Autodesk Inventor part; units mm, degrees
ref_plane "Płaszczyzna konstrukcyjna1" through (0, -12, 0) normal (0, 0, -1) x (-1, 0, 0)
ref_plane "Płaszczyzna konstrukcyjna2" through (0, -10, -2.2657) normal (1, 0, 0) x (0, 0, -1)
ref_plane "YZ Plane" through (0, 0, 0) normal (1, 0, 0) x (0, 1, 0)
sketch "Szkic1" plane through (0, 0, 0) normal (0, 1, 0) x (-1, 0, 0)
  circle A0 centre (0, 0) radius 12.5
  circle A1 centre (0, 0) radius 10
  dimension "d0" = 20
  dimension "d2" = 25
extrude "Wyciągnięcie proste1" add sketch "Szkic1" along normal blind 5
ref_plane "Płaszczyzna konstrukcyjna1" through (0, -12, 0) normal (0, 0, -1) x (-1, 0, 0)
sketch "Szkic5" plane through (0, -12, 0) normal (0, 0, -1) x (-1, 0, 0)
  line L0 (12.5, 17) -> (-12.5, 17)
  line L1 (0, 17) -> (-12.5, 17)
  line L2 (-12.5, 17) -> (-12.5, 19.375)
  line L3 (-12.5, 19.375) -> (0, 19.375)
  line L4 (0, 19.375) -> (0, 17)
  line L5 (0, 19.375) -> (-9.5, 19.375)
  line L6 (-9.5, 19.375) -> (-9.5, 21.875)
  line L7 (-9.5, 21.875) -> (0, 21.875)
  line L8 (0, 21.875) -> (0, 19.375)
  line L9 (0, 21.875) -> (-12.5, 21.875)
  line L10 (-12.5, 21.875) -> (-12.5, 24.25)
  line L11 (-12.5, 24.25) -> (0, 24.25)
  line L12 (0, 24.25) -> (0, 21.875)
  line L13 (0, 24.25) -> (-9.5, 24.25)
  line L14 (-9.5, 24.25) -> (-9.5, 26.75)
  line L15 (-9.5, 26.75) -> (0, 26.75)
  line L16 (0, 26.75) -> (0, 24.25)
  line L17 (0, 26.75) -> (-12.5, 26.75)
  line L18 (-12.5, 26.75) -> (-12.5, 29.125)
  line L19 (-12.5, 29.125) -> (0, 29.125)
  line L20 (0, 29.125) -> (0, 26.75)
  line L21 (0, 29.125) -> (-9.5, 29.125)
  line L22 (-9.5, 29.125) -> (-9.5, 31.625)
  line L23 (-9.5, 31.625) -> (0, 31.625)
  line L24 (0, 31.625) -> (0, 29.125)
  line L25 (0, 31.625) -> (-12.5, 31.625)
  line L26 (-12.5, 31.625) -> (-12.5, 34)
  line L27 (-12.5, 34) -> (0, 34)
  line L28 (0, 34) -> (0, 31.625)
  line L29 (-12.5, 12) -> (-12.5, 17) construction
  line L30 (-12.5, 12) -> (-12.5, 17) construction
  line L31 (-12.5, 12) -> (12.5, 12) construction
  point P0 (0, 12)
  dimension "d13" = 2.5
  dimension "d17" = 22
  dimension "d18" = 3
revolve "Obrót1" add sketch "Szkic5" angle 360 about axis through (0, 12.25, 0) along (0, -1, 0)
sketch "Szkic7" plane through (0, 19.625, 0) normal (0, -1, 0) x (1, 0, 0)
  circle A0 centre (0, 0) radius 9.5
  circle A1 centre (0, 9.5) radius 1.65
  circle A2 centre (0, 0) radius 10
  circle A3 centre (0, 0) radius 9.5
  circle A4 centre (-9.5, 0) radius 1.65
  circle A5 centre (0, -9.5) radius 1.65
  circle A6 centre (9.5, 0) radius 1.65
  circle A7 centre (6.7175, -6.7175) radius 0.9
  circle A8 centre (6.7175, 6.7175) radius 0.9
  circle A9 centre (-6.7175, 6.7175) radius 0.9
  circle A10 centre (-6.7175, -6.7175) radius 0.9
  line L0 (6.7175, 6.7175) -> (0, 0) construction
  line L1 (0, 0) -> (-6.7175, 6.7175) construction
  circle A11 centre (0, 0) radius 12.5 construction
  line L2 (0, 0) -> (-6.7175, -6.7175) construction
  line L3 (0, 0) -> (6.7175, -6.7175) construction
  line L4 (17.5, 0) -> (-17.5, 0) construction
  dimension "d23" = 45
  dimension "d24" = 45
  dimension "d25" = 3.3
  dimension "d47" = 1.8
extrude "Wyciągnięcie proste6" cut sketch "Szkic7" along normal up to surface (12.25 mm away) contours A0 A6 | A0 A6 A2 | A8 A0 | A0 A8 A2 | A6 A2 | A7 A2 A0 | A0 A7 | A2 A8 | A7 A2 | A1 A0 | A0 A1 A2 | A5 A2 A0 | A0 A5 | A2 A1 | A5 A2 | A9 A0 | A0 A9 A2 | A10 A2 A0 | A0 A10 | A2 A9 | A10 A2 | A4 A0 | A0 A4 A2 | A2 A4
sketch "Szkic8" plane through (0, -12, 0) normal (0, 0, -1) x (-1, 0, 0)
  line L0 (-1.65, 24.25) -> (1.65, 24.25)
  line L1 (-1.65, 29.125) -> (-1.65, 21.875)
  line L2 (1.65, 24.25) -> (-1.65, 24.25)
  line L3 (-1.65, 24.25) -> (-1.65, 26.751)
  line L4 (-1.65, 26.751) -> (1.65, 26.751)
  line L5 (1.65, 26.751) -> (1.65, 24.25)
  point P0 (0, 12)
  point P1 (-1.6438, 24.25)
  point P2 (1.6438, 24.25)
extrude "Wyciągnięcie proste7" cut sketch "Szkic8" along normal through all both and the other way through all
sketch "Szkic9" plane through (0, 5, 0) normal (0, -1, 0) x (1, 0, 0)
  line L0 (0, 0) -> (-3.4352, 0)
  line L1 (-3.4352, 0) -> (-3.4352, -2.2657)
  line L2 (-3.4352, -2.2657) -> (0, -2.2657)
  line L3 (0, -2.2657) -> (0, 0)
  dimension "d30" = 3.4352
  dimension "d31" = 2.2658
extrude "Wyciągnięcie proste8" add sketch "Szkic9" along normal blind 15
ref_plane "Płaszczyzna konstrukcyjna2" through (0, -10, -2.2657) normal (1, 0, 0) x (0, 0, -1)
sketch "Szkic10" plane through (0, -10, 0) normal (0, -1, 0) x (1, 0, 0)
  line L0 (0, 0) -> (-3.4352, 0)
  line L1 (-3.4352, -2.2657) -> (0, -2.2657)
  line L2 (0, 0) -> (-3.4352, 0)
  line L3 (-3.4352, 0) -> (-3.4352, -2.2657)
  line L4 (-3.4352, -2.2657) -> (0, -2.2657)
  line L5 (0, -2.2657) -> (0, 0)
extrude "Wyciągnięcie proste9" cut sketch "Szkic10" against normal up to surface (15 mm away)
sketch "Szkic11" plane through (0, -10, -2.2657) normal (1, 0, 0) x (0, 0, -1)
  line L0 (-3.9095, 22.25) -> (-3.9095, 24.75)
  line L1 (-0.622, 22.25) -> (-0.622, 24.75)
  line L2 (-3.9095, 22.25) -> (-0.622, 22.25)
  line L3 (-0.622, 22.25) -> (-0.622, 24.75)
  line L4 (-0.622, 24.75) -> (-3.9095, 24.75)
  line L5 (-3.9095, 24.75) -> (-3.9095, 22.25)
  point P0 (-2.2657, 10)
extrude "Wyciągnięcie proste10" cut sketch "Szkic11" along normal through all both and the other way through all
sketch "Szkic12" plane through (0, 22, 0) normal (0, 1, 0) x (1, 0, 0)
  line L0 (0, 0) -> (-4.4901, 4.4901) construction
  line L1 (0, 0) -> (0, 6.35) construction
  line L2 (0, 0) -> (-4.4901, -4.4901) construction
  line L3 (0, 0) -> (4.4901, -4.4901) construction
  line L4 (0, 0) -> (4.4901, 4.4901) construction
  circle A0 centre (0, 0) radius 6.35 construction
  circle A1 centre (0, 0) radius 12.5 construction
  point P0 (-4.4901, -4.4901)
  dimension "d48" = 45
  dimension "d49" = 12.7
hole "Otwór1" at (-4.4901, 22, -4.4901) at (-4.4901, 22, 4.4901) at (4.4901, 22, 4.4901) at (4.4901, 22, -4.4901) direction (0, -1, 0) diameter 3.4 end through all countersink diameter 6.9 countersink angle 89.954
properties part number "Koło"
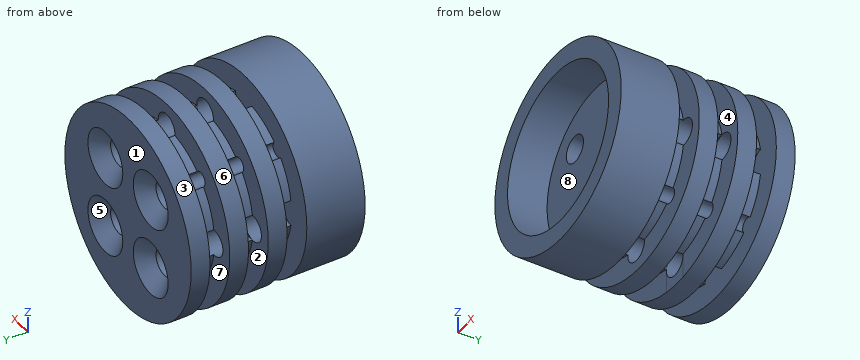
Could you check a few things on this model? Use its own coordinates, in mm. Face numbers are marked on the shaded views. A direction names the side the tool comes from. Round coordinates to 2 decimals unless told otherwise and drop trailing zeros. Order: outer loops, then holes, each group sorted by start corner. A loop starts at its lowest first (then second) coordinate and runs counter-clockwise, first axis right, second up.
Q1. Imagine slicing it at C-C, the plane y = 4. List the corners of the cut face in (x, z) for me, then the cut area to 3 significant figures.
Geometry says:
outline: circle Ø25 at (0, 0); hole circle Ø20 at (0, 0)
area: 177 mm2
Q2. Imagine slicing it at D-D, the plane z = -4.5. State how many separate pieces and enclosed holes the cut face has, then the cut area to 3 significant figures.
Geometry says:
separate pieces: 3
enclosed holes: 1
area: 244 mm2
Q3. Imagine slicing it at B-B, the plane y = 9.25. List the corners of the cut face in (x, z) for me.
Geometry says:
outline: (-9.36, -1.64) arc R9.5 ccw to (-7.32, -6.05) arc R0.9 cw to (-6.05, -7.32) arc R9.5 ccw to (-1.64, -9.36) arc R1.65 cw to (1.64, -9.36) arc R9.5 ccw to (6.05, -7.32) arc R0.9 cw to (7.32, -6.05) arc R9.5 ccw to (9.36, -1.64) arc R1.65 cw to (9.36, 1.64) arc R9.5 ccw to (7.32, 6.05) arc R0.9 cw to (6.05, 7.32) arc R9.5 ccw to (1.64, 9.36) arc R1.65 cw to (-1.64, 9.36) arc R9.5 ccw to (-6.05, 7.32) arc R0.9 cw to (-7.32, 6.05) arc R9.5 ccw to (-9.36, 1.64) arc R1.65 cw to start; hole circle Ø3.4 at (-4.49, -4.49); hole circle Ø3.4 at (-4.49, 4.49); hole circle Ø3.4 at (4.49, -4.49); hole circle Ø3.4 at (4.49, 4.49)
Q4. Thinking about a two-plate mould opening in Y: for the marked faces 1, 2 and 3, which applies, released by +Y, released by -Y, zero draft, split by the parting line, or undercut?
Geometry says:
face 1: released by +Y
face 2: undercut
face 3: zero draft
Q5. I'm going to push flat-ended pins straight in: P1, Ø6, axis at y = 6.5, z = 0.5, coming from the -X side; P2, Ø1.3, axis at y = 14, z = -4.5, coming from the +X side; P3, Ø1, axis at y = 19, z = -4, coming from the +X side; P4, Ø12, axis at x = -6.5, y = 18, coming from the +Z side. Where does each tip first touch, or does it pass through?
Geometry says:
P1: stops at x = -12.5
P2: stops at x = 8.68
P3: stops at x = 8.83
P4: stops at z = 12.49
Q6. Please list where these lines run through material, in increasing order: probe 1 along Y at (x, z) = (-3.75, 9.5) (3 decimals); probe 2 along Z at (x, y) = (0, 16.05); probe 3 along X at (y, z) = (13.5, -5.5).
Geometry says:
probe 1: y = 0 to 7.375, 9.875 to 12.25, 14.75 to 17.125, 19.625 to 22
probe 2: z = -12.5 to -11.15, -7.85 to 7.85, 11.15 to 12.5
probe 3: x = -7.75 to -5.86, -3.12 to -1.65, 1.65 to 3.12, 5.86 to 7.75
Q7. Which directions (+Z, -Z, +X, -X, +Y, -Y) give clear straight access to the entire face, cutting with the end or side of a thin tool? Please do the marked faces 4, 5, 6, 7 and 8.
Geometry says:
face 4: +X
face 5: +Y
face 6: +Y, -Y
face 7: none
face 8: -Y
